Geometry: final body of the model. Coordinates: model frame, mm. A direction names the side the tool comes from. Give positions to 0.01 mm unless a question says otherwise; leave off trailing zeros. Loops run counter-clockwise (first coordinate to the right, second up) from the corner with the lowest first, then second, coordinate; pieces in that order, holes last. Notation, with made-up numbers: (-13.75, -10) - (-2.75, -10) arc R24 ccw to (-2.75, 24) - close; hole circle Ø6 at (-37, 1.25). An arc over 180 degrees is marked (long way). Answer in a Markdown table with one row per item.
from build123d import *

# Parameters (mm, degrees)
F2_R     = 42.5
F2_R_2   = 75
F2_R_3   = 15
F3_DEPTH = 25


# Not quite as in the source:
# - ends of sketch curves that miss each other by under 0.0002 mm in the source are joined


with BuildPart() as f1:
    # F0 (on Front) → F1 (revolve)
    with BuildSketch(Plane.XZ):
        with BuildLine():
            Line((-221.3601278806, 0), (0, 0))
            Line((0, 0), (0, 6))
            Line((0, 6), (-221.3601278806, 6))
            ThreePointArc((-221.3601278806, 6), (-222.7368362926, 6.5492520372), (-223.3573858774, 7.8953281437))
            Line((-223.3573858774, 7.8953281437), (-223.9088928554, 18.4186876499))
            ThreePointArc((-223.9088928554, 18.4186876499), (-226.3910925279, 23.8029949681), (-231.8979291334, 26))
            Line((-231.8979291334, 26), (-250, 26))
            Line((-250, 26), (-250, 20))
            Line((-250, 20), (-231.8979291334, 20))
            ThreePointArc((-231.8979291334, 20), (-230.521219982, 19.450748742), (-229.9006700639, 18.1046719125))
            Line((-229.9006700639, 18.1046719125), (-229.3491641587, 7.5813123501))
            ThreePointArc((-229.3491641587, 7.5813123501), (-226.8669644862, 2.1970050319), (-221.3601278806, 0))
        make_face()
    revolve(axis=Axis((0, 0, 34.008089453), (0, 0, 1)))

    # F2 (on Top) → F3 (cut)
    with BuildSketch(Plane.XY):
        with Locations((-110, -110)):
            Circle(F2_R)
        with Locations((110, -110)):
            Circle(F2_R)
        with Locations((110, 110)):
            Circle(F2_R)
        with Locations((-110, 110)):
            Circle(F2_R)
        Circle(F2_R_2)
        with Locations((0, -175)):
            Circle(F2_R_3)
        with Locations((0, 175)):
            Circle(F2_R_3)
    extrude(amount=F3_DEPTH, mode=Mode.SUBTRACT)


solid = f1.part
Q1. Cut plane A-A (x = 0). Give the number of separate pieces and of enclosed holes in the cut face, and give its area (3 significant figures).
Check values:
| item | result |
|---|---|
| separate pieces | 4 |
| enclosed holes | 0 |
| area | 1,920 mm² |
Q2. Cut plane B-B (y = 0). Output: boundary loops of the cut face in (x, z), and give its area (3 significant figures).
Check values:
| item | result |
|---|---|
| outline | (-250, 20) - (-231.9, 20) arc R2 cw to (-229.9, 18.1) - (-229.35, 7.58) arc R8 ccw to (-221.36, 0) - (-75, 0) - (-75, 6) - (-221.36, 6) arc R2 cw to (-223.36, 7.9) - (-223.91, 18.42) arc R8 ccw to (-231.9, 26) - (-250, 26) - close; (75, 0) - (221.36, 0) arc R8 ccw to (229.35, 7.58) - (229.9, 18.1) arc R2 cw to (231.9, 20) - (250, 20) - (250, 26) - (231.9, 26) arc R8 ccw to (223.91, 18.42) - (223.36, 7.9) arc R2 cw to (221.36, 6) - (75, 6) - close |
| area | 2,280 mm² |
Q3. First-contact query: pin 1 (12 mm diameter, centred on x = 132, y = 157, fed in from +Z); pin 2 (6 mm diameter, centred on x = 123.5, z = 16.5, fed in from -Y); pin 3 (4 mm diameter, centred on x = 168, z = 3.5, fed in from +Y). Flat tips, straight axial feed; report the tip coordinate or a pass-through.
Check values:
| item | result |
|---|---|
| pin 1 | z = 6 |
| pin 2 | y = -195.7 |
| pin 3 | y = 156.82 |
Q4. Reachability of faces 1 (the cylindrical face through (-69.463, 122.766, 2.958)), 2 (the flat face through (-221, 73, 20)) from +Z, -Z, +X, -X, +Y, -Y: full face, straight path, thin tool, end or side. Return the list, or none.
Check values:
| item | result |
|---|---|
| face 1 | +Z, -Z |
| face 2 | -Z |
Q5. Draft query along X for faces 3 (the flat face through (-3, 95, 6)), 4 (the cylindrical face through (249.76, -10.99, 22.96)), 5 (the flat face through (221, 73, 26)). Return one class per face: pulls with the +X half, pulls with the -X half, needs draft (parallel to the pull), parting line crosses it, or undercut.
Check values:
| item | result |
|---|---|
| face 3 | undercut |
| face 4 | parting line crosses it |
| face 5 | needs draft |
Q6. Material intervals for line 1 along Y through (x, z) = (0, 1.65); line 2 along Y through (x, z) = (-110, 4.2); line 3 along Y through (x, z) = (0, 1.8), sorted ascending.
Check values:
| item | result |
|---|---|
| line 1 | -226.23 to -190, -160 to -75, 75 to 160, 190 to 226.23 |
| line 2 | -200.17 to -152.5, -67.5 to 67.5, 152.5 to 200.17 |
| line 3 | -226.42 to -190, -160 to -75, 75 to 160, 190 to 226.42 |
